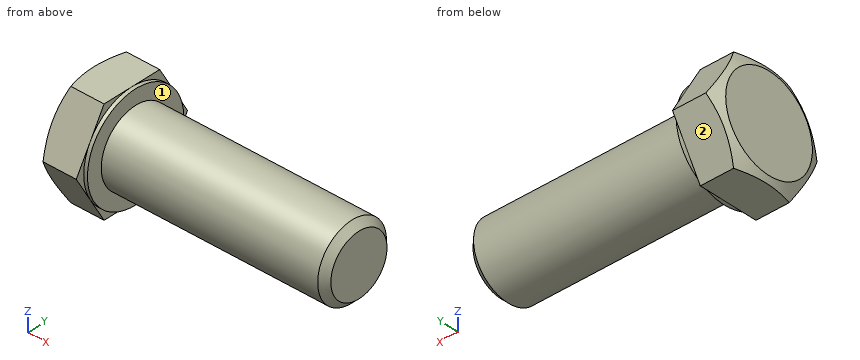
Autodesk Inventor part; units mm, degrees
ref_plane "Work Plane1" through (1.525, 0, 0) normal (0, 0, 1) x (1, 0, 0)
ref_plane "YZ Plane" through (0, 0, 0) normal (1, 0, 0) x (0, 1, 0)
ref_plane "XZ Plane" through (0, 0, 0) normal (0, 1, 0) x (-1, 0, 0)
sketch "Эскиз1" plane through (0, 0, 0) normal (0, 0, 1) x (1, 0, 0)
  line L0 (0, 7) -> (0, 5)
  line L1 (1.5, 5) -> (30, 5)
  line L2 (30, 5) -> (30, 0)
  line L3 (30, 0) -> (-0.5001, 0)
  line L4 (-6.6001, 0) -> (36.1, 0)
  line L5 (-0.5001, 0) -> (-0.5001, 7)
  line L6 (-0.5001, 7) -> (0, 7)
  line L7 (1.5, 5) -> (0.5797, 5)
  line L8 (0.5797, 5) -> (0, 5)
  line L9 (0, -1.4) -> (0, 8.4)
  dimension "d0" = 30
  dimension "d1" = 28.5
  dimension "d2" = 10
  dimension "d9" = 0.5001
  dimension "d10" = 14
  dimension "d13" = 0.9203
  dimension "d14" = 10
revolve "Базовый элемент" add sketch "Эскиз1" angle 360 about axis through (30, 0, 0) along (-1, 0, 0)
sketch "Эскиз2" plane through (-0.5001, 0, 0) normal (-1, 0, 0) x (0, 0, 1)
  line L0 (0, 8.0829) -> (7, 4.0415)
  line L1 (7, 4.0415) -> (7, -4.0415)
  line L2 (7, -4.0415) -> (0, -8.0829)
  line L3 (0, -8.0829) -> (-7, -4.0415)
  line L4 (-7, -4.0415) -> (-7, 4.0415)
  line L5 (-7, 4.0415) -> (0, 8.0829)
  point P0 (0, 0)
  point P1 (0, 0)
  dimension "d11" = 14
extrude "С головкой" add sketch "Эскиз2" along normal blind 5.5
sketch "Эскиз4" plane through (0, 0, 0) normal (0, 0, 1) x (1, 0, 0)
  line L0 (-6.0001, 6.3) -> (-6.0001, 8.0829)
  line L1 (-6.0001, 8.0829) -> (-4.9707, 8.0829)
  line L2 (-4.9707, 8.0829) -> (-6.0001, 6.3)
  line L3 (-7.1001, 0) -> (0.5999, 0)
  line L4 (-0.5001, 8.0829) -> (-6.0001, 8.0829)
  line L5 (-6.0001, 4.0415) -> (-6.0001, 8.0829)
  dimension "d5" = 30
  dimension "d19" = 12.6
revolve "Фаска1" cut sketch "Эскиз4" angle 360 about axis through (-10, 0, 0) along (1, 0, 0)
thread "Резьба"
chamfer "Фаска2" distance 0.9202 distance2 0.9203 1 edges at (30, -5, 0) measured on face at (30, -0.2009, 0.1054)
ref_plane "Work Plane1" through (1.525, 0, 0) normal (0, 0, 1) x (1, 0, 0)
equation "\"d0\" = NLG"
equation "\"d1\" = GEL"
equation "\"d2\" = GD"
equation "\"d10\" = SD2"
equation "\"d14\" = BDM"
equation "\"d11\" = SW"
equation "\"d3\" = KOH - SD"
equation "\"d5\" = ANG1"
equation "\"d19\" = SW0"
equation "\"d15\" = GEL"
equation "\"d6\" = -0.5 * SPD + 0.5 * GD"
equation "\"NLG\" = 30"
equation "\"GD\" = NND"
equation "\"BDM\" = NND"
equation "\"KOH\" = 6"
equation "\"GEL\" = 28.5"
equation "\"SW\" = 14"
equation "\"SW0\" = 12.6"
equation "\"SPD\" = NND - 1.2269 * PTC"
equation "\"SD2\" = SW"
equation "\"SD\" = 0.5"
equation "\"ANG1\" = 30deg"
equation "\"GAL\" = 0.61345 * PTC"
equation "\"GUL\" = 0.61345 * PTC"
equation "\"RR\" = 0.1"
equation "\"GD1\" = THREADDIA - 1.2269 * PTC"
equation "\"TOA\" = 30deg"
equation "\"PTC\" = 1.5"
equation "\"E0\" = 1.155 * SW"
properties part number "Болт M10-6gx30 ГОСТ 7808-70" material "Сталь, мягкая"
Geometry: final body of the model. Coordinates: model frame, mm. Face numbers are marked on the shaded views. A direction names the side the tool comes from. Give positions to 0.01 mm unless a question says otherwise; leave off trailing zeros. Loops run counter-clockwise (first coordinate to the right, second up) from the corner with the lowest first, then second, coordinate; pieces in that order, holes last. Notation, with made-up numbers: (6.25, 83) -> (20.25, 83) arc R9 ccw to (20.25, 91) -> close; hole circle Ø3 at (19, -25.75). An arc over 180 degrees is marked (long way). Return JSON: item names as keys, results as strings.
Item 1: Line query: line 1 (X direction, y = 3.5, z = 4.25); line 2 (Z direction, x = 8.5, y = 3.75); line 3 (Z direction, x = 27.5, y = 1.25). Output: solid intervals per line, ascending.
Filled in:
{"line 1": "-6 to 0", "line 2": "-3.31 to 3.31", "line 3": "-4.84 to 4.84"}
Item 2: Pin query (flat end, axial travel): P1, Ø4, axis at y = 4, z = 5, coming from the +X side; P2, Ø4, axis at y = 4.5, z = -5, coming from the +X side; P3, Ø1.5, axis at y = -5, z = -2.5, coming from the +X side. Return the tip coordinate at first contact, or that it passes through.
Filled in:
{"P1": "x = 29.68", "P2": "x = 29.35", "P3": "x = 29.24"}
Item 3: Access query for the marked faces 1 and 2. Directions: +Z, -Z, +X, -X, +Y, -Y. A direction counts if a zero-diameter tool reaches every point of the face in a straight line with its end or side. Return the directions, or none.
Filled in:
{"face 1": "+X", "face 2": "-Z, +X, -X, +Y"}
Item 4: Section A-A, the plane x = 18. Output: boundary loops of the cut face in (y, z), plus the area to 3 significant figures.
Filled in:
{"outline": "circle Ø10 at (0, 0)", "area": "78.5 mm^2"}
